Input: part model. Units: mm. Frame: model coordinates. Face numbers are marked on the shaded views. A direction names the side the tool comes from. Give positions to 0.01 mm unless a question says otherwise; leave off trailing zeros. Order: outer loops, then holes, each group sorted by start corner. A loop starts at its lowest first (then second) coordinate and runs counter-clockwise, first axis right, second up. Notation, with made-up numbers: M -33,61.25 L 22,61.25 A23 ccw 22,93.25 Z; hole C 85.5,34.25 d2. An arc over 180 degrees is marked long. Use a Markdown table: item, result.
from build123d import *

# Parameters (mm, degrees)
SKETCH_W     = 15.49
SKETCH_H     = 21.33
PAD_DEPTH    = 8.13
SKETCH001_W  = 17.55
SKETCH001_H  = 27.48
PAD001_DEPTH = 2
SKETCH002_W  = 10
SKETCH002_H  = 3
PAD002_DEPTH = 7.5
PAD003_DEPTH = 10
FILLET_R     = 1
FILLET001_R  = 1
FILLET002_R  = 1.5


with BuildPart() as part:
    # Sketch → Pad (new body)
    with BuildSketch(Plane.XY):
        Rectangle(SKETCH_W, SKETCH_H)
    extrude(amount=PAD_DEPTH)

    # Sketch001 (on Face6 of Pad) → Pad001 (join)
    with BuildSketch(Plane.XY.offset(8.13)):
        Rectangle(SKETCH001_W, SKETCH001_H)
    extrude(amount=PAD001_DEPTH)

    # Sketch002 (on Face5 of Pad001) → Pad002 (join)
    with BuildSketch(Plane.XY.offset(10.13)):
        Rectangle(SKETCH002_W, SKETCH002_H)
    extrude(amount=PAD002_DEPTH)

    # Sketch003 (on Face14 of Pad002) → Pad003 (join)
    with BuildSketch(Plane(origin=(-5, 0, 0), x_dir=(0, -1, 0), z_dir=(-1, 0, 0))):
        with BuildLine():
            ThreePointArc((1.5, 17.63), (6.562473, 12.154115), (13.74, 10.13))
            Line((1.5, 10.13), (13.74, 10.13))
            Line((1.5, 17.63), (1.5, 10.13))
        make_face()
    pad003 = extrude(amount=-PAD003_DEPTH)

    # Mirrored: Pad003 across Sketch003 V_Axis
    add(pad003.mirror(Plane(origin=(-5, 0, 0), x_dir=(-1, 0, 0), z_dir=(0, -1, 0))))

    # Fillet
    fillet_edges = [part.edges().sort_by_distance(p)[0] for p in [
        (-8.775, 0, 10.13),
        (-6.8875, -13.74, 10.13),
        (-6.8875, 13.74, 10.13),
        (6.8875, 13.74, 10.13),
        (6.8875, -13.74, 10.13),
        (8.775, 0, 10.13),
    ]]
    fillet(fillet_edges, radius=FILLET_R)

    # Fillet001
    fillet001_edges = [part.edges().sort_by_distance(p)[0] for p in [
        (0, -13.74, 10.13),
        (0, 13.74, 10.13),
    ]]
    fillet(fillet001_edges, radius=FILLET001_R)

    # Fillet002
    fillet002_edges = [part.edges().sort_by_distance(p)[0] for p in [
        (0, 1.5, 17.63),
        (0, -1.5, 17.63),
    ]]
    fillet(fillet002_edges, radius=FILLET002_R)


solid = part.part
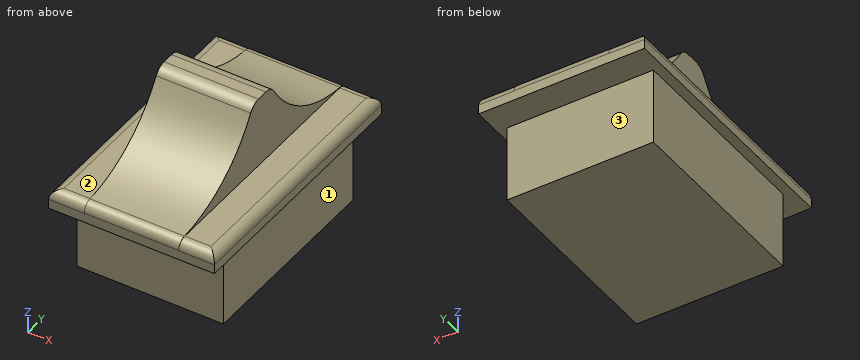
1) Material intervals for line 1 (Y direction, x = -1.5, z = 1.5) (3 decimals); line 2 (Z direction, x = 6.25, y = 1); line 3 (X direction, y = 0, z = 12.25), sorted ascending. Write a range as from..to.
Response values:
| item | result |
|---|---|
| line 1 | y = -10.665..10.665 |
| line 2 | z = 0..10.13 |
| line 3 | x = -5..5 |
2) Cut plane C-C on x = -7. Return loops of the section in (y, z) (3 decimals), and give its area (3 significant figures).
Response values:
| item | result |
|---|---|
| outline | M -13.74,8.13 L -10.665,8.13 L -10.665,0 L 10.665,0 L 10.665,8.13 L 13.74,8.13 L 13.74,9.13 A1 ccw 12.74,10.13 L -12.74,10.13 A1 ccw -13.74,9.13 Z |
| area | 228 mm² |
3) Cut plane D-D on z = 6.25. Return loops of the section in (x, y) (3 decimals).
Response values:
| item | result |
|---|---|
| outline | M -7.745,-10.665 L 7.745,-10.665 L 7.745,10.665 L -7.745,10.665 Z |
4) Cut plane B-B on y = -0.25. Return loops of the section in (x, z) (3 decimals), and give its area (3 significant figures).
Response values:
| item | result |
|---|---|
| outline | M -8.775,8.13 L -7.745,8.13 L -7.745,0 L 7.745,0 L 7.745,8.13 L 8.775,8.13 L 8.775,9.13 A1 ccw 7.775,10.13 L 5,10.13 L 5,17.63 L -5,17.63 L -5,10.13 L -7.775,10.13 A1 ccw -8.775,9.13 Z |
| area | 236 mm² |
5) Cut plane A-A on x = 1.5. Return loops of the section in (y, z) (3 decimals), and give its area (3 significant figures).
Response values:
| item | result |
|---|---|
| outline | M -13.74,8.13 L -10.665,8.13 L -10.665,0 L 10.665,0 L 10.665,8.13 L 13.74,8.13 L 13.74,9.164 A1 ccw 12.808,10.162 A13.738 cw 1.905,16.892 A1.5 ccw 0.613,17.63 L -0.613,17.63 A1.5 ccw -1.905,16.892 A13.738 cw -12.808,10.162 A1 ccw -13.74,9.164 Z |
| area | 303 mm² |
6) Reachability of the marked faces 1, 2 and 3 from +Z, -Z, +X, -X, +Y, -Y: full face, straight path, thin tool, end or side. Return the list, or none.
Response values:
| item | result |
|---|---|
| face 1 | -Z, +X, +Y, -Y |
| face 2 | +Z, -X, +Y, -Y |
| face 3 | -Z, +X, -X, +Y |
7) First-contact query: pin 1 Ø2 at (y, z) = (4, 4) entering from -X (3 decimals); pin 2 Ø6.5 at (x, z) = (-2.5, 2) entering from +Y (3 decimals); pin 3 Ø4 at (x, z) = (-4, 15.5) entering from +Y. Flat tips, straight axial feed; report the tip coordinate or a pass-through.
Response values:
| item | result |
|---|---|
| pin 1 | stops at x = -7.745 |
| pin 2 | stops at y = 10.665 |
| pin 3 | stops at y = 4.73 |
